Verification items for the finished model (mm, model axes). A direction names the side the tool comes from. Coordinates: 2 decimals unless noted, no trailing zeros. Order: outer loops, then holes, each group sorted by start corner. A loop starts at its lowest first (then second) coordinate and runs counter-clockwise, first axis right, second up. Notation, with made-up numbers: (-7.5, 71.25) -> (17.5, 71.25) arc R14 cw to (17.5, 94.25) -> close; hole circle Ø9 at (11.25, 24.25). An arc over 180 degrees is marked (long way). Write each question's results on one line, items separated by ' | '. Start each with the question number.
(1) Cross-section at B-B on z = 0.5. Enter the section's corners in (x, y) (3 decimals).
(2) Cross-section at A-A on x = 9.5. Enter the section's corners in (y, z) (3 decimals), and give its area (3 significant figures).
(3) Thickness scan on probe 1 along Y at (x, z) = (-9.5, 1.8) (3 decimals); probe 2 along X at (y, z) = (-0.95, -2); probe 3 along X at (y, z) = (0.8, 2.75). Record the ranges inside material, lowest first. Write a range as [from, to].
(4) Set-up check for faces 5 (the flat face through (-12, 0, 1)), 6 (the flat face through (-4, 0, 2)), 7 (the flat face through (7.5, 0, -1)), 8 (the flat face through (-7.5, 0, -1)): record each of +Z, -Z, +X, -X, +Y, -Y from which the full face is reachable in a straight line by a thin tool's end or side.
(5) Draft check along X on faces 1 (the flat face through (4, 0, 2)), 2 (the cylindrical face through (0.16, 0.04, -9.5)), 3 (the flat face through (-11.3, 0, 0)), 4 (the cylindrical face through (-11.123, 0.071, 1.479)). Enter one of: +X half, -X half, draft (parallel to the pull), parting line (faces both ways), or undercut.
(6) Cross-section at D-D on z = -5.5. Enter the section's corners in (x, y).
(7) Go/stop test with flat-tipped pins: pin 1 (3 mm diameter, centred on x = -9.5, y = 0, fed in from +Z); pin 2 (2 mm diameter, centred on x = -10, y = -0.5, fed in from -Z); pin 3 (1 mm diameter, centred on y = -0.5, z = -2, fed in from -X); pin 4 (1 mm diameter, centred on y = -1, z = -1.5, fed in from +X). Record where each tip stops, or that it passes through.
(8) Cross-section at C-C on y = 0. Enter the section's corners in (x, z) (3 decimals), and give its area (3 significant figures).
```python
from build123d import *

# Parameters (mm, degrees)
F0_W     = 24
F0_H     = 6
F0_R     = 1.625
F1_DEPTH = 3
F3_DEPTH = 6
F5_DEPTH = 6.001


with BuildPart() as f1:
    # F0 (on Top) → F1 (new body)
    with BuildSketch(Plane.XY):
        Rectangle(F0_W, F0_H)
        with Locations((-9.5, 0)):
            Circle(F0_R, mode=Mode.SUBTRACT)
        with Locations((9.5, 0)):
            Circle(F0_R, mode=Mode.SUBTRACT)
    extrude(amount=F1_DEPTH)

    # F2 (on face) → F3 (join)
    with BuildSketch(Plane(origin=(0, 3, 0), x_dir=(-1, 0, 0), z_dir=(0, 1, 0))):
        with BuildLine():
            Line((-7.5, 0), (-7.5, -2))
            ThreePointArc((-7.5, -2), (0, -9.5), (7.5, -2))
            Line((7.5, -2), (7.5, 0))
            Line((7.5, 0), (4.582575695, 0))
            ThreePointArc((4.582575695, 0), (4.8945315647, -0.9784517816), (5, -2))
            ThreePointArc((5, -2), (-1.0215482184, -6.8945315647), (-4.582575695, 0))
            Line((-4.582575695, 0), (-7.5, 0))
        make_face()
    extrude(amount=-F3_DEPTH)

    # F4 (on face) → F5 (cut, through all)
    with BuildSketch(Plane.XZ.offset(3)):
        with BuildLine():
            Line((-4, 3), (-4, 1))
            ThreePointArc((-4, 1), (-2.2360679775, 2.472135955), (0, 3))
            Line((0, 3), (-4, 3))
        make_face()
        with BuildLine():
            Line((-4.582575695, 0), (-4, 0))
            Line((-4, 0), (-4, 1))
            ThreePointArc((-4, 1), (-4.3203184362, 0.5169125154), (-4.582575695, 0))
        make_face()
        with BuildLine():
            Line((-4, 1), (-4, 0))
            Line((-4, 0), (4, 0))
            Line((4, 0), (4, 1))
            ThreePointArc((4, 1), (2.2360679775, 2.472135955), (0, 3))
            ThreePointArc((0, 3), (-2.2360679775, 2.472135955), (-4, 1))
        make_face()
        with BuildLine():
            Line((4, 3), (0, 3))
            ThreePointArc((0, 3), (2.2360679775, 2.472135955), (4, 1))
            Line((4, 1), (4, 3))
        make_face()
        with BuildLine():
            Line((4, 1), (4, 0))
            Line((4, 0), (4.582575695, 0))
            ThreePointArc((4.582575695, 0), (4.3203184362, 0.5169125154), (4, 1))
        make_face()
    extrude(amount=-F5_DEPTH, mode=Mode.SUBTRACT)


solid = f1.part
```
Results are:
1) outline: (-12, -3) -> (-4.33, -3) -> (-4.33, 3) -> (-12, 3) -> close; (4.33, -3) -> (12, -3) -> (12, 3) -> (4.33, 3) -> close; hole circle Ø3.25 at (-9.5, 0); hole circle Ø3.25 at (9.5, 0)
2) outline: (-3, 0) -> (-1.625, 0) -> (-1.625, 3) -> (-3, 3) -> close; (1.625, 0) -> (3, 0) -> (3, 3) -> (1.625, 3) -> close | area: 8.25 mm2
3) probe 1: y = [-3, -1.625], [1.625, 3] | probe 2: x = [-7.5, -5], [5, 7.5] | probe 3: x = [-12, -10.91], [-8.09, -4], [4, 8.09], [10.91, 12]
4) face 5: +Z, -Z, -X, +Y, -Y | face 6: +Z, +Y, -Y | face 7: -Z, +X, +Y, -Y | face 8: -Z, -X, +Y, -Y
5) face 1: undercut | face 2: parting line | face 3: draft | face 4: undercut
6) outline: (-6.63, -3) -> (-3.57, -3) -> (-3.57, 3) -> (-6.63, 3) -> close; (3.57, -3) -> (6.63, -3) -> (6.63, 3) -> (3.57, 3) -> close
7) pin 1: passes through | pin 2: stops at z = 0 | pin 3: stops at x = -7.5 | pin 4: stops at x = 7.5
8) outline: (-12, 0) -> (-11.125, 0) -> (-11.125, 3) -> (-12, 3) -> close; (-7.875, 0) -> (-7.5, 0) -> (-7.5, -2) arc R7.5 ccw to (7.5, -2) -> (7.5, 0) -> (7.875, 0) -> (7.875, 3) -> (4, 3) -> (4, 1) arc R5 cw (long way) to (-4, 1) -> (-4, 3) -> (-7.875, 3) -> close; (11.125, 0) -> (12, 0) -> (12, 3) -> (11.125, 3) -> close | area: 87.5 mm2
